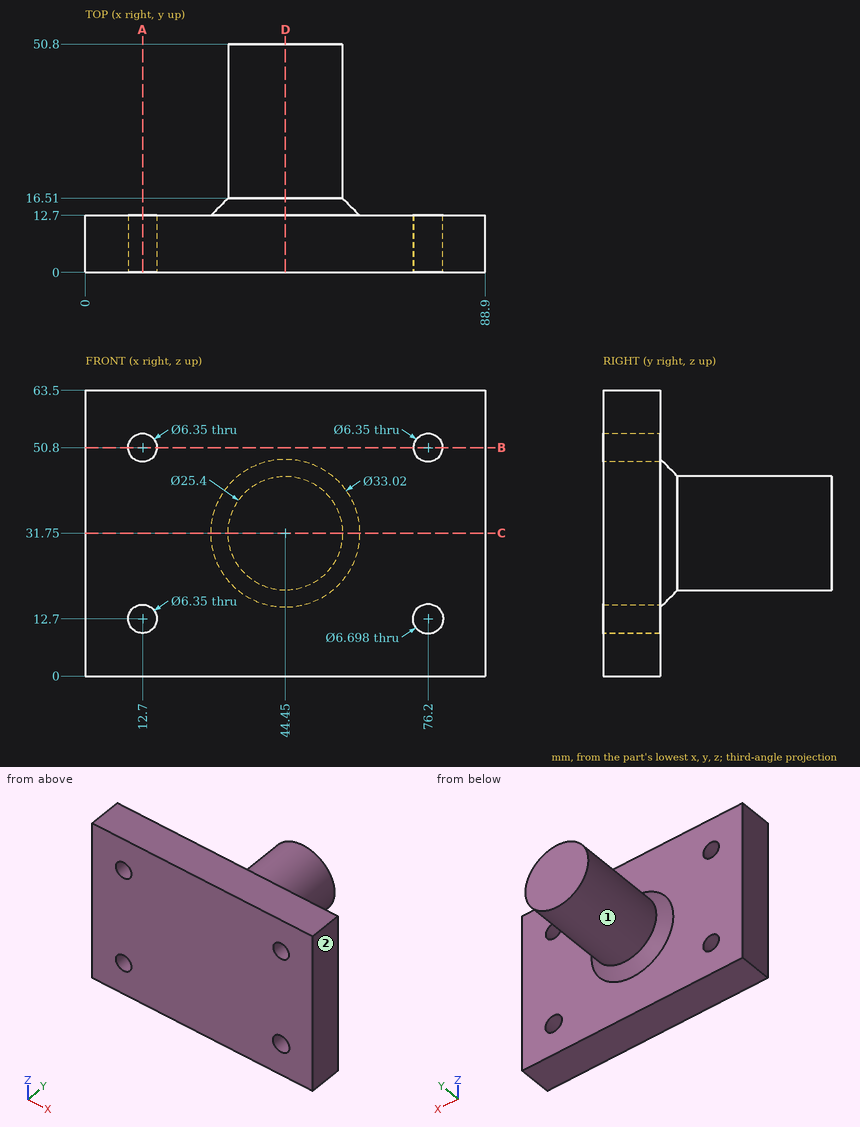
Geometry check sheet. Reference: drawing and pictorial views, mm from the part's lowest x, y, z. A direction names the side the tool comes from. Round coordinates to 2 decimals unless told otherwise and drop trailing zeros. Loops run counter-clockwise (first coordinate to the right, second up) from the corner with the lowest first, then second, coordinate; pieces in that order, holes last. Notation, with made-up numbers: (61, -33.75) -> (90, -33.75) arc R33 ccw to (90, 0.25) -> close; hole circle Ø4 at (35.25, 48.5). An arc over 180 degrees is marked (long way). Answer as a JSON object with one key per item and string values. Group by question number.
Item 1: Cross-section at D-D, the plane x = 44.45. Record the cut outline in (y, z), plus the area to 3 significant figures.
Item 2: Cross-section at B-B, the plane z = 50.8. Record the cut outline in (x, y) (1 decimal), plus the area to 3 significant figures.
Item 3: Depth check by flat-ended pin: pin 1 Ø7.5 at (x, z) = (76.2, 12.7) entering from -Y; pin 2 Ø3 at (x, y) = (45, 23) entering from +Z; pin 3 Ø1.5 at (y, z) = (45.5, 41.5) entering from -X; pin 4 Ø3 at (y, z) = (14.5, 53.5) entering from +X. Enter the tip coordinate at first touch or a pass-through.
Item 4: Cross-section at A-A, the plane x = 12.7. Record the cut outline in (y, z) (1 decimal).
Item 5: Thickness scan on line 1 along X through (y, z) = (9.25, 50.8) (1 decimal); line 2 along X through (y, z) = (9, 50); line 3 along Y through (x, z) = (61.5, 24). Record the ranges inside material, lowest first.
Item 6: Cross-section at C-C, the plane z = 31.75. Record the cut outline in (x, y).
Item 7: Set-up check for the marked faces 1 and 2: record each of +Z, -Z, +X, -X, +Y, -Y from which the full face is reachable in a straight line by a thin tool's end or side.
Determined:
{
 "1": {"outline": "(0, 0) -> (12.7, 0) -> (12.7, 15.24) -> (16.51, 19.05) -> (50.8, 19.05) -> (50.8, 44.45) -> (16.51, 44.45) -> (12.7, 48.26) -> (12.7, 63.5) -> (0, 63.5) -> close", "area": "1,790 mm²"},
 "2": {"outline": "(0, 0) -> (9.5, 0) -> (9.5, 12.7) -> (0, 12.7) -> close; (15.9, 0) -> (73, 0) -> (73, 12.7) -> (15.9, 12.7) -> close; (79.4, 0) -> (88.9, 0) -> (88.9, 12.7) -> (79.4, 12.7) -> close", "area": "968 mm²"},
 "3": {"pin 1": "stops at y = 0", "pin 2": "stops at z = 44.45", "pin 3": "stops at x = 35.49", "pin 4": "passes through"},
 "4": {"outline": "(0, 0) -> (12.7, 0) -> (12.7, 9.5) -> (0, 9.5) -> close; (0, 15.9) -> (12.7, 15.9) -> (12.7, 47.6) -> (0, 47.6) -> close; (0, 54) -> (12.7, 54) -> (12.7, 63.5) -> (0, 63.5) -> close"},
 "5": {"line 1": "x = 0 to 9.5, 15.9 to 73, 79.4 to 88.9", "line 2": "x = 0 to 9.63, 15.77 to 73.13, 79.27 to 88.9", "line 3": "y = 0 to 12.7"},
 "6": {"outline": "(0, 0) -> (88.9, 0) -> (88.9, 12.7) -> (60.96, 12.7) -> (57.15, 16.51) -> (57.15, 50.8) -> (31.75, 50.8) -> (31.75, 16.51) -> (27.94, 12.7) -> (0, 12.7) -> close"},
 "7": {"face 1": "+Y", "face 2": "+Z, -Z, +X, +Y, -Y"}
}
